Geometry: final body of the model. Coordinates: model frame, mm. Give positions to 0.01 mm unless a question says otherwise; leave off trailing zeros. Write each loop counter-clockwise with the first axis right and the second up, starting at its lowest first coordinate (ties: lowest second). Pieces come first, ordered by that corner, then holes. Notation, with made-up numbers: (24, -19) -> (43, -19) arc R31 cw to (43, 13) -> close; hole circle Ø8 at (39, 80.25). An arc over 180 degrees is marked (long way). Answer in a Markdown table with one row per item. Add a question column.
from build123d import *

# Parameters (mm, degrees)
SKETCH1_R           = 2.265
BOSS_EXTRUDE1_DEPTH = 3
CUT_EXTRUDE3_DEPTH  = 3
SKETCH8_W           = 6.5
SKETCH8_H           = 20
CUT_EXTRUDE4_DEPTH  = 3
BOSS_EXTRUDE4_DEPTH = 3
FILLET1_R           = 0.6


with BuildPart() as part:
    # Sketch1 → Boss-Extrude1 (new body)
    with BuildSketch(Plane(origin=(0, 0, 0), x_dir=(1, 0, 0), z_dir=(0, 1, 0))):
        with BuildLine():
            Line((0, -4.265), (0, -58.735))
            ThreePointArc((0, -58.735), (-3.015810422, -66.015810422), (4.265, -63))
            Line((4.265, -63), (87.735, -63))
            ThreePointArc((87.735, -63), (95.015810422, -66.015810422), (92, -58.735))
            Line((92, -58.735), (92, -4.265))
            ThreePointArc((92, -4.265), (95.015810422, 3.015810422), (87.735, 0))
            Line((87.735, 0), (4.265, 0))
            ThreePointArc((4.265, 0), (-3.015810422, 3.015810422), (0, -4.265))
        make_face()
        with Locations(Location((0, 0, 0), (0, 0, 270))):
            Circle(SKETCH1_R, mode=Mode.SUBTRACT)
        with Locations(Location((92, 0, 0), (0, 0, 270))):
            Circle(SKETCH1_R, mode=Mode.SUBTRACT)
        with Locations(Location((92, -63, 0), (0, 0, 270))):
            Circle(SKETCH1_R, mode=Mode.SUBTRACT)
        with Locations(Location((0, -63, 0), (0, 0, 270))):
            Circle(SKETCH1_R, mode=Mode.SUBTRACT)
    extrude(amount=BOSS_EXTRUDE1_DEPTH)

    # Sketch6 → Cut-Extrude3 (cut)
    with BuildSketch(Plane(origin=(0, 3, 0), x_dir=(1, 0, 0), z_dir=(0, 1, 0))):
        with BuildLine():
            Line((18, -30), (22.5, -30))
            Line((22.5, -30), (22.5, -25.5))
            ThreePointArc((22.5, -25.5), (24, -24), (25.5, -25.5))
            Line((25.5, -25.5), (25.5, -30))
            Line((25.5, -30), (30, -30))
            ThreePointArc((30, -30), (31.5, -31.5), (30, -33))
            Line((30, -33), (25.5, -33))
            Line((25.5, -33), (25.5, -37.5))
            ThreePointArc((25.5, -37.5), (24, -39), (22.5, -37.5))
            Line((22.5, -37.5), (22.5, -33))
            Line((22.5, -33), (18, -33))
            ThreePointArc((18, -33), (16.5, -31.5), (18, -30))
        make_face()
        with BuildLine():
            Line((74, -30), (69.5, -30))
            Line((69.5, -30), (69.5, -25.5))
            ThreePointArc((69.5, -25.5), (68, -24), (66.5, -25.5))
            Line((66.5, -25.5), (66.5, -30))
            Line((66.5, -30), (62, -30))
            ThreePointArc((62, -30), (60.5, -31.5), (62, -33))
            Line((62, -33), (66.5, -33))
            Line((66.5, -33), (66.5, -37.5))
            ThreePointArc((66.5, -37.5), (68, -39), (69.5, -37.5))
            Line((69.5, -37.5), (69.5, -33))
            Line((69.5, -33), (74, -33))
            ThreePointArc((74, -33), (75.5, -31.5), (74, -30))
        make_face()
    extrude(amount=-CUT_EXTRUDE3_DEPTH, mode=Mode.SUBTRACT)

    # Sketch8 → Cut-Extrude4 (cut)
    with BuildSketch(Plane(origin=(0, 3, 0), x_dir=(1, 0, 0), z_dir=(0, 1, 0))):
        with Locations((3.25, -31.5)):
            Rectangle(SKETCH8_W, SKETCH8_H)
    extrude(amount=-CUT_EXTRUDE4_DEPTH, mode=Mode.SUBTRACT)

    # Sketch9 → Boss-Extrude4 (add)
    with BuildSketch(Plane(origin=(0, 3, 0), x_dir=(1, 0, 0), z_dir=(0, 1, 0))):
        with BuildLine():
            Line((0, -21.5), (-2.5, -21.5))
            ThreePointArc((-2.5, -21.5), (-2.853553391, -21.353553391), (-3, -21))
            Line((-3, -21), (-3, -15.746058789))
            ThreePointArc((-3, -15.746058789), (-2.931958048, -15.555807734), (-2.758696908, -15.451857033))
            Line((-2.758696908, -15.451857033), (0, -14.901462701))
            Line((0, -14.901462701), (0, -21.5))
        make_face()
        with BuildLine():
            Line((0, -41.5), (0, -48.098537299))
            Line((0, -48.098537299), (-2.758696908, -47.548142967))
            ThreePointArc((-2.758696908, -47.548142967), (-2.931958048, -47.444192266), (-3, -47.253941211))
            Line((-3, -47.253941211), (-3, -42))
            ThreePointArc((-3, -42), (-2.853553391, -41.646446609), (-2.5, -41.5))
            Line((-2.5, -41.5), (0, -41.5))
        make_face()
    extrude(amount=-BOSS_EXTRUDE4_DEPTH)

    # Fillet1
    fillet1_edges = [part.edges().sort_by_distance(p)[0] for p in [
        (6.5, 1.5, 21.5),
        (6.5, 1.5, 41.5),
        (0, 1.5, 14.901462701),
        (4.265, 1.5, 0),
        (87.735, 1.5, 0),
        (92, 1.5, 4.265),
        (92, 1.5, 58.735),
        (87.735, 1.5, 63),
        (4.265, 1.5, 63),
        (0, 1.5, 58.735),
        (0, 1.5, 4.265),
        (0, 1.5, 48.098537299),
    ]]
    fillet(fillet1_edges, radius=FILLET1_R)


solid = part.part
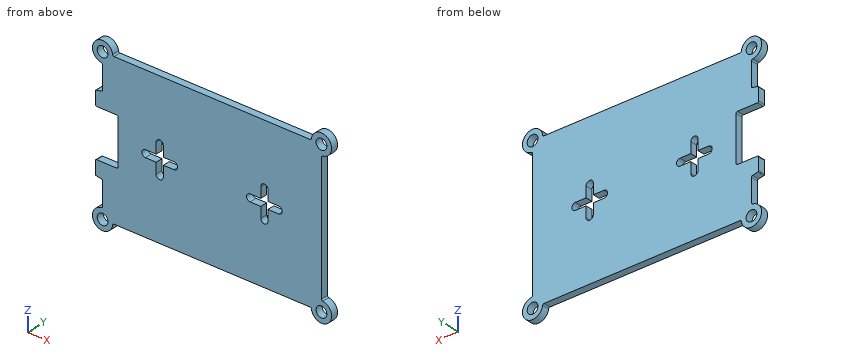
Q1. Section C-C on y = 0.65. Count the separate pieces of the cut face and the enclosed holes in it, and give its area (3 significant figures).
Q2. Section A-A on x = 26.5. Return loops of the section in (y, z).
Q3. Section B-B on z = 29. Return loops of the section in (x, y), and give its area (4 significant figures).
Q4. Contact query for flat-ended pins moving along their axis: pin 1 Ø1 at (x, y) = (40.5, 1.5) entering from +Z; pin 2 Ø1.5 at (y, z) = (1.5, 18) entering from -X; pin 3 Ø1.5 at (y, z) = (1.5, 28) entering from +X. Output: stop coordinate, or through.
Q5. Section D-D on z = 11.5. Return loops of the section in (x, y), and give its area (3 significant figures).
Q6. Line query: probe 1 along Z at (x, y) = (19, 1.6); probe 2 along Z at (x, y) = (39.5, 1.8); probe 3 along X at (y, z) = (1.75, 17). Output: solid intervals per line, ascending. Write a range as from..to.
Checks:
| question | item | result |
|---|---|---|
| 1 | separate pieces | 1 |
| 1 | enclosed holes | 6 |
| 1 | area | 5,660 mm^2 |
| 2 | outline | (0, 0) -> (3, 0) -> (3, 30) -> (0, 30) -> close; (0, 33) -> (3, 33) -> (3, 63) -> (0, 63) -> close |
| 3 | outline | (6.5, 0) -> (22.5, 0) -> (22.5, 3) -> (6.5, 3) -> close; (25.5, 0) -> (66.5, 0) -> (66.5, 3) -> (25.5, 3) -> close; (69.5, 0) -> (92, 0) -> (92, 3) -> (69.5, 3) -> close |
| 3 | area | 238.5 mm^2 |
| 4 | pin 1 | z = 63 |
| 4 | pin 2 | x = -3 |
| 4 | pin 3 | x = 92 |
| 5 | outline | (0, 0) -> (92, 0) -> (92, 3) -> (0, 3) -> close |
| 5 | area | 276 mm^2 |
| 6 | probe 1 | 0..30, 33..63 |
| 6 | probe 2 | 0..63 |
| 6 | probe 3 | -3..92 |
